The listing builds one solid part. Answer for the finished solid, in the listing's coordinates (mm). Face numbers are marked on the shaded views. A direction names the side the tool comes from. Give positions to 0.01 mm unless a question says otherwise; leave off trailing zeros. Order: outer loops, then holes, each group sorted by start corner. A loop starts at its lowest first (then second) coordinate and runs counter-clockwise, first axis right, second up.
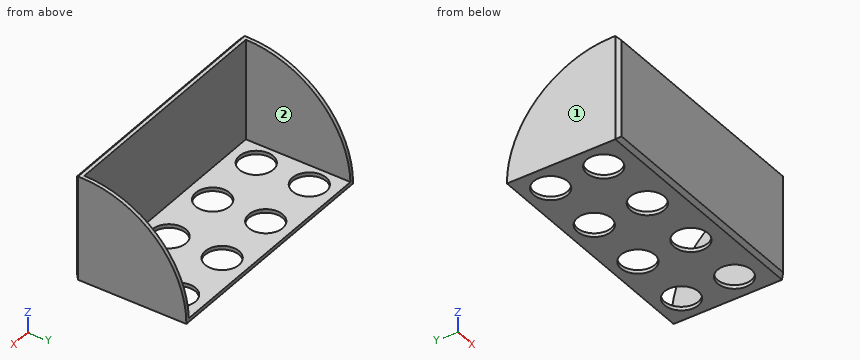
```python
from build123d import *

# Parameters (mm, degrees)
F0_W     = 82.55
F0_H     = 36.068
F0_R     = 5.842
F1_DEPTH = 1.27
F2_W     = 1.27
F2_H     = 36.068
F3_DEPTH = 50.8
F5_DEPTH = 101.6
F6_W     = 80.01
F6_H     = 34.798
F7_DEPTH = 2.54
F9_SIZE  = 1.27


with BuildPart() as f1:
    # F0 (on Top) → F1 (new body)
    with BuildSketch(Plane.XY):
        with Locations((41.275, 18.034)):
            Rectangle(F0_W, F0_H)
        with Locations((8.89, 8.89)):
            Circle(F0_R, mode=Mode.SUBTRACT)
        with Locations((30.48, 8.89)):
            Circle(F0_R, mode=Mode.SUBTRACT)
        with Locations((52.07, 8.89)):
            Circle(F0_R, mode=Mode.SUBTRACT)
        with Locations((73.66, 8.89)):
            Circle(F0_R, mode=Mode.SUBTRACT)
        with Locations((8.89, 27.178)):
            Circle(F0_R, mode=Mode.SUBTRACT)
        with Locations((30.48, 27.178)):
            Circle(F0_R, mode=Mode.SUBTRACT)
        with Locations((52.07, 27.178)):
            Circle(F0_R, mode=Mode.SUBTRACT)
        with Locations((73.66, 27.178)):
            Circle(F0_R, mode=Mode.SUBTRACT)
    extrude(amount=F1_DEPTH)

    # F2 (on face) → F3 (join)
    with BuildSketch(Plane.XY.offset(1.27)):
        with Locations((0.635, 18.034)):
            Rectangle(F2_W, F2_H)
        with Locations((81.915, 18.034)):
            Rectangle(F2_W, F2_H)
    extrude(amount=F3_DEPTH)

    # F4 (on face) → F5 (cut)
    with BuildSketch(Plane(origin=(0, 0, 0), x_dir=(0, -1, 0), z_dir=(-1, 0, 0))):
        with BuildLine():
            Line((-36.068, 52.07), (-36.068, 0))
            ThreePointArc((-36.068, 0), (-25.5039273838, 25.5039273838), (0, 36.068))
            Line((0, 36.068), (0, 52.07))
            Line((0, 52.07), (-36.068, 52.07))
        make_face()
    extrude(amount=-F5_DEPTH, mode=Mode.SUBTRACT)


with BuildPart() as f7:
    # F6 (on face) → F7 (new body)
    with BuildSketch(Plane.XZ):
        with Locations((41.275, 18.669)):
            Rectangle(F6_W, F6_H)
        Polygon((0, 36.068), (0, 0), (82.55, 0), (82.55, 36.068), (81.28, 36.068), (81.28, 1.27), (1.27, 1.27), (1.27, 36.068), align=None)
    extrude(amount=F7_DEPTH)


with BuildPart() as f1_1:
    add(f1.part)

    # F8: union F7
    add(f7.part)

    # F9
    f9_edges = [f1_1.edges().sort_by_distance(p)[0] for p in [
        (82.55, -2.54, 18.034),
        (41.275, -2.54, 36.068),
        (41.275, -2.54, 0),
        (0, -2.54, 18.034),
    ]]
    chamfer(f9_edges, length=F9_SIZE)


solid = f1_1.part
```
1) Find section D-D (x = 39.5). Write down the section's boundary in (y, z).
Geometry says:
outline: (-2.54, 1.27) - (-1.27, 0) - (36.07, 0) arc R36.07 ccw to (36.05, 1.27) - (0, 1.27) - (0, 36.07) - (-1.27, 36.07) - (-2.54, 34.8) - close
2) Find section A-A (x = 52.07). Write down the section's boundary in (y, z).
Geometry says:
outline: (-2.54, 1.27) - (-1.27, 0) - (3.05, 0) - (3.05, 1.27) - (0, 1.27) - (0, 36.07) - (-1.27, 36.07) - (-2.54, 34.8) - close; (14.73, 0) - (21.34, 0) - (21.34, 1.27) - (14.73, 1.27) - close; (33.02, 0) - (36.07, 0) arc R36.07 ccw to (36.05, 1.27) - (33.02, 1.27) - close
3) A tool of negligible diameter and unlimited length cuts with its end or side. For the marked faces 1 and 2, from which of +Z, -Z, +X, -X, +Y, -Y can it reach the whole face along a straight path? Write none if from no direction.
Geometry says:
face 1: +Z, -Z, -X, +Y, -Y
face 2: +Z, +Y
4) Find section C-C (z = 16). Write down the section's boundary in (x, y), then the cut area to 3 significant figures.
Geometry says:
outline: (0, -1.27) - (1.27, -2.54) - (81.28, -2.54) - (82.55, -1.27) - (82.55, 32.32) - (81.28, 32.32) - (81.28, 0) - (1.27, 0) - (1.27, 32.32) - (0, 32.32) - close
area: 290 mm2
5) Find section B-B (y = 28.5). Write down the section's boundary in (x, z).
Geometry says:
outline: (0, 0) - (3.2, 0) - (3.2, 1.27) - (1.27, 1.27) - (1.27, 22.11) - (0, 22.11) - close; (14.58, 0) - (24.79, 0) - (24.79, 1.27) - (14.58, 1.27) - close; (36.17, 0) - (46.38, 0) - (46.38, 1.27) - (36.17, 1.27) - close; (57.76, 0) - (67.97, 0) - (67.97, 1.27) - (57.76, 1.27) - close; (79.35, 0) - (82.55, 0) - (82.55, 22.11) - (81.28, 22.11) - (81.28, 1.27) - (79.35, 1.27) - close
6) Straight lines are drawn through the part: probe 1 along X at (y, z) = (6.5, 27); probe 2 along Y at (x, z) = (73.66, 0.85); probe 3 along Y at (x, z) = (52.07, 0.5). For each, find the intervals that lie inside material, in ascending order.
Geometry says:
probe 1: x = 0 to 1.27, 81.28 to 82.55
probe 2: y = -2.12 to 3.05, 14.73 to 21.34, 33.02 to 36.06
probe 3: y = -1.77 to 3.05, 14.73 to 21.34, 33.02 to 36.06
7) Given P1, Ø8, axis at x = 34.5, y = 19.5, coming from the +Z side; P2, Ø1, axis at x = 62.5, z = 5.5, coming from the +Y side, each flat-ended and moving along its own axis, determine where each tip first touches the part or whether it passes through.
Geometry says:
P1: stops at z = 1.27
P2: stops at y = 0
